Build history of the part. All positions in model axes, mm. A direction names the side the tool comes from. Round coordinates to 2 decimals unless told otherwise and drop trailing zeros. Write each loop counter-clockwise with the first axis right and the second up, starting at its lowest first coordinate (ties: lowest second). Pieces come first, ordered by that corner, then holes. Notation, with made-up numbers: (-12, 3) - (36, 3) arc R36 cw to (36, 39) - close; hole circle Ø9 at (78, -12). An arc over 180 degrees is marked (long way). One line per question, with ' | ' between items.
from build123d import *

# Parameters (mm, degrees)
BOSS_EXTRUDE1_DEPTH = 5
SKETCH2_R           = 5
BOSS_EXTRUDE2_DEPTH = 20
SKETCH3_R           = 2.5
BOSS_EXTRUDE3_DEPTH = 5


with BuildPart() as part:
    # Sketch1 → Boss-Extrude1 (new body)
    with BuildSketch(Plane.XY):
        with BuildLine():
            Line((0, 14.259541246), (20.176972809, 21.540123656))
            ThreePointArc((20.176972809, 21.540123656), (42.215740985, 7.597057881), (20.176972809, -6.346007893))
            Line((20.176972809, -6.346007893), (0, 0))
            ThreePointArc((0, 0), (-5.564259015, 7.129770623), (0, 14.259541246))
        make_face()
    extrude(amount=BOSS_EXTRUDE1_DEPTH)

    # Sketch2 → Boss-Extrude2 (add)
    with BuildSketch(Plane.XY.offset(5)):
        with Locations((26.785740985, 7.597057881)):
            Circle(SKETCH2_R)
    extrude(amount=BOSS_EXTRUDE2_DEPTH)

    # Sketch3 → Boss-Extrude3 (add)
    with BuildSketch(Plane(origin=(0, 0, 0), x_dir=(-1, 0, 0), z_dir=(0, 0, -1))):
        with Locations((-1.785740985, 7.129770623)):
            Circle(SKETCH3_R)
    extrude(amount=BOSS_EXTRUDE3_DEPTH)


solid = part.part
Q1. Drop flat-ended pins along their axis: pin 1 (3 mm diameter, centred on y = 2.5, z = 17, fed in from +X); pin 2 (2 mm diameter, centred on y = 3, z = 1, fed in from -X); pin 3 (6 mm diameter, centred on x = 30.5, z = 0, fed in from -Y). Give the stop position or say it passes through.
Found:
pin 1: x = 30.26 | pin 2: x = -4.86 | pin 3: y = -7.82
Q2. Which spindle directions (+Z, -Z, +X, -X, +Y, -Y) get a long thin tool onto all of the face, cutting with end or side? Do faces 1 (the cylindrical face through (31.555, 9.099, 14.86)), 2 (the cylindrical face through (-5.563, 6.993, 2.465)), 3 (the cylindrical face through (-0.6, 7.88, -2.46)). Say none if no direction does.
Found:
face 1: +Z | face 2: +Z, -Z, -X | face 3: -Z
Q3. Saw through at D-D, the plane y = 19. List the corners of the cut face in (x, z).
Found:
outline: (13.14, 0) - (37.18, 0) - (37.18, 5) - (13.14, 5) - close
Q4. Saw through at C-C, the plane z = 12. List the corners of the cut face in (x, y), then the cut area to 3 significant figures.
Found:
outline: circle Ø10 at (26.79, 7.6) | area: 78.5 mm^2
Q5. Saw through at B-B, the plane x = 25. List the corners of the cut face in (y, z).
Found:
outline: (-7.73, 0) - (22.92, 0) - (22.92, 5) - (12.27, 5) - (12.27, 25) - (2.93, 25) - (2.93, 5) - (-7.73, 5) - close
Q6. Pull direction Z, two halves, no side cores. Call faces 4 (the flat face through (27, 8, 25)), 5 (the flat face through (2, 7, -5)), 6 (the flat face through (10.23, -3.217, 2.465)): +Z half, -Z half, draft (parallel to the pull), parting line (faces both ways), or undercut.
Found:
face 4: +Z half | face 5: -Z half | face 6: draft
Q7. Saw through at A-A, the plane y = 6.5. List the corners of the cut face in (x, z).
Found:
outline: (-5.54, 0) - (-0.63, 0) - (-0.63, -5) - (4.21, -5) - (4.21, 0) - (42.18, 0) - (42.18, 5) - (31.66, 5) - (31.66, 25) - (21.91, 25) - (21.91, 5) - (-5.54, 5) - close
Q8. Drill centre lines: L1, parallel to Z at x = 5.5, y = 3; L2, parallel to X at y = 10, z = 18; L3, parallel to X at y = 7, z = 21. Where is each one in solid material? Low to high. Write a range as from..to.
Found:
L1: 0..5 | L2: 22.4..31.17 | L3: 21.82..31.75
